Geometry check sheet. Reference: the model listing, model coordinates, mm. Face numbers are marked on the shaded views. Round coordinates to 2 decimals unless told otherwise and drop trailing zeros. Order: outer loops, then holes, each group sorted by start corner. A loop starts at its lowest first (then second) coordinate and runs counter-clockwise, first axis right, second up.
(1) Sectioned sample at C-C (y = -2.5). Record the boundary of the cut face in (x, z), plus the area to 3 significant figures.
(2) Release check for a two-part mould opening along Z. For the marked faces 1, 2, 3 and 4 record: +Z half, -Z half, draft (parallel to the pull), parting line (faces both ways), or undercut.
(3) Go/stop test with a flat-tipped pin: pin 1 (2 mm diameter, centred on x = 0, z = 0, fed in from +Y). Record where the tip stops, or that it passes through.
(4) Sectioned sample at A-A (z = 0). Record the boundary of the cut face in (x, y), plus the area to 4 significant figures.
(5) Material ranges on line 1 along X through (y, z) = (0, 2.85), recorded low to high.
from build123d import *

# Parameters (mm, degrees)
SKETCH_1_W      = 10
SKETCH_1_H      = 10
EXTRUDE_1_DEPTH = 5
HOLE_WIZARD_1_D = 2.5
HOLE_WIZARD_2_D = 2.5
HOLE_WIZARD_3_D = 2.5


with BuildPart() as part:
    # 草图1 → 凸台-拉伸1 (new, symmetric)
    with BuildSketch(Plane(origin=(0, 0, 0), x_dir=(1, 0, 0), z_dir=(0, 1, 0))):
        Rectangle(SKETCH_1_W, SKETCH_1_H)
    extrude(amount=EXTRUDE_1_DEPTH, both=True)

    # Hole Wizard 1 (through all)
    with Locations(Plane(origin=(0, 5, 0), x_dir=(1, 0, 0), z_dir=(0, 1, 0))):
        with Locations((0, 0)):
            Hole(HOLE_WIZARD_1_D / 2)

    # Hole Wizard 2 (through all)
    with Locations(Plane(origin=(5, 0, 0), x_dir=(0, 0, -1), z_dir=(1, 0, 0))):
        with Locations((0, 0)):
            Hole(HOLE_WIZARD_2_D / 2)

    # Hole Wizard 3 (through all)
    with Locations(Plane.XY.offset(5)):
        with Locations((0, 0)):
            Hole(HOLE_WIZARD_3_D / 2)


solid = part.part
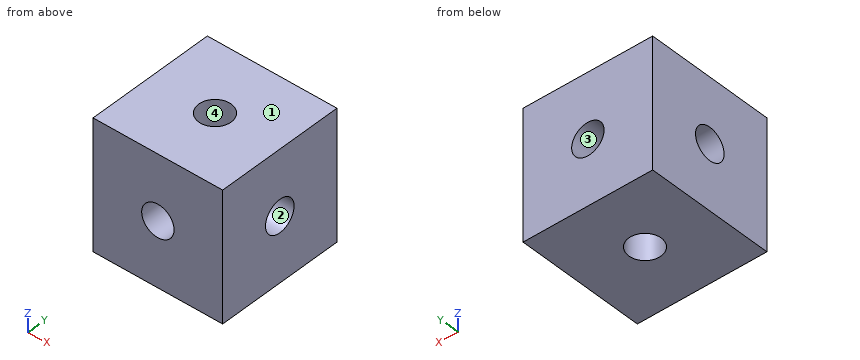
Answer below:
1. outline: (-5, -5) - (5, -5) - (5, 5) - (-5, 5) - close; hole circle Ø2.5 at (0, 0)
1. area: 95.1 mm2
2. face 1: +Z half
2. face 2: undercut
2. face 3: undercut
2. face 4: draft
3. pin 1: passes through
4. outline: (-5, -5) - (-1.25, -5) - (-1.25, -1.25) - (-5, -1.25) - close; (-5, 1.25) - (-1.25, 1.25) - (-1.25, 5) - (-5, 5) - close; (1.25, -5) - (5, -5) - (5, -1.25) - (1.25, -1.25) - close; (1.25, 1.25) - (5, 1.25) - (5, 5) - (1.25, 5) - close
4. area: 56.25 mm2
5. line 1: x = -5 to -1.25, 1.25 to 5
